The drawing under review shows one solid part. Ordinate dimensions are in mm from its lowest x, y, z. Round coordinates to 2 decimals unless told otherwise and drop trailing zeros. Order: outer loops, then holes, each group sorted by start corner. A loop starts at its lowest first (then second) coordinate and runs counter-clockwise, first axis right, second up. Notation, with made-up numbers: M -35,-17.5 L -15,-17.5 A10 ccw -15,-12.5 Z; hole C -5,78.25 d5. An arc over 180 degrees is marked long. Use a Markdown table: item, result.
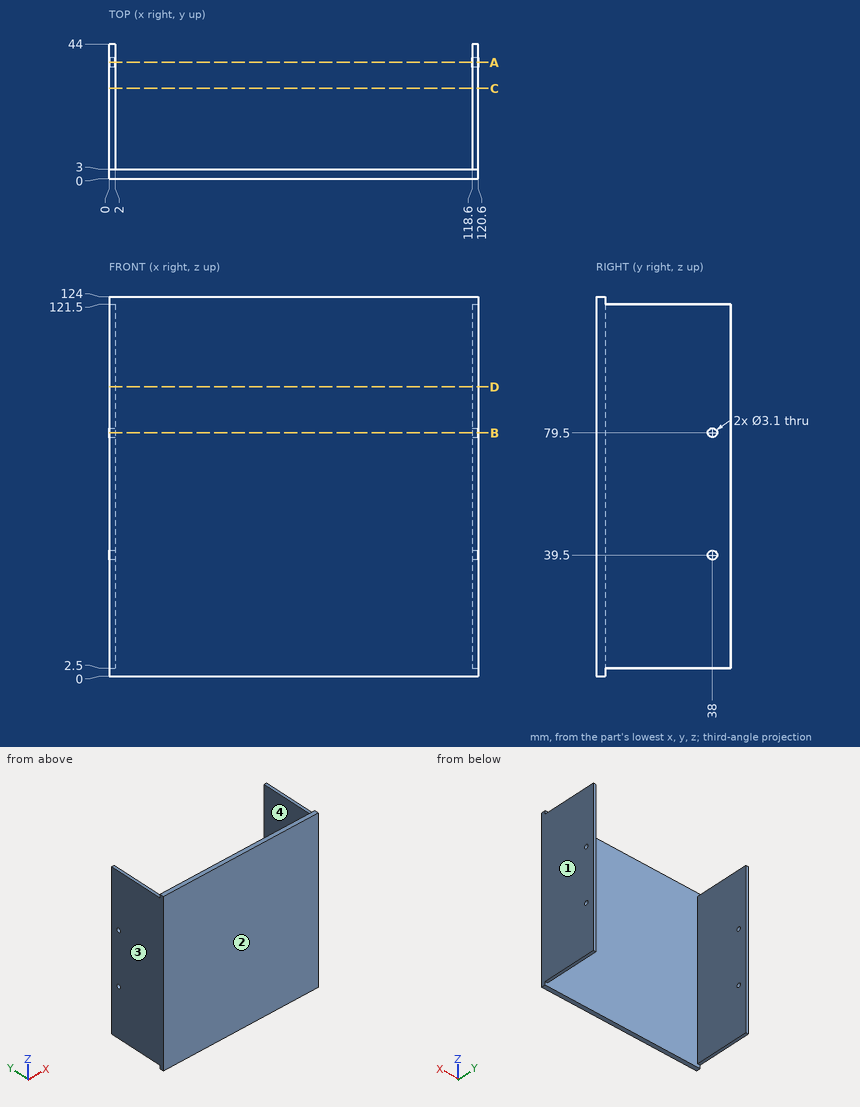
Q1. Wall thickness on line 1 along X through (y, z) = (28, 50); line 2 along Y through (x, z) = (0.65, 39.5); line 3 along Y through (x, z) = (51, 29): over which ranges is each line inside the solid? List them lowest first. Write a range as [from, to].
Determined:
| item | result |
|---|---|
| line 1 | x = [0, 2], [118.6, 120.6] |
| line 2 | y = [0, 36.45], [39.55, 44] |
| line 3 | y = [0, 3] |
Q2. Clearance check with flat-ended pins moving along their axes: pin 1 (2.5 mm diameter, centred on y = 38, z = 79.5, fed in from +X); pin 2 (1 mm diameter, centred on x = 120, y = 31.5, fed in from +Z); pin 3 (2 mm diameter, centred on x = 120, y = 32.5, fed in from -Z). State where each tip first meets the part, or that it passes through.
Determined:
| item | result |
|---|---|
| pin 1 | passes through |
| pin 2 | stops at z = 121.5 |
| pin 3 | stops at z = 2.5 |
Q3. Add section D-D (z = 94.5). Write out the cut boundary in (x, y).
Determined:
| item | result |
|---|---|
| outline | M 0,0 L 120.6,0 L 120.6,44 L 118.6,44 L 118.6,3 L 2,3 L 2,44 L 0,44 Z |
Q4. Draft analysis for pull direction X (two halves, no side actions). For the marked faces 1, 2, 3 and 4, state which applies: pulls with the +X half, pulls with the -X half, needs draft (parallel to the pull), parting line crosses it, or undercut.
Determined:
| item | result |
|---|---|
| face 1 | pulls with the +X half |
| face 2 | needs draft |
| face 3 | pulls with the -X half |
| face 4 | undercut |
Q5. Add section B-B (z = 79.5). Write out the cut boundary in (x, y).
Determined:
| item | result |
|---|---|
| outline | M 0,0 L 120.6,0 L 120.6,36.45 L 118.6,36.45 L 118.6,3 L 2,3 L 2,36.45 L 0,36.45 Z; M 0,39.55 L 2,39.55 L 2,44 L 0,44 Z; M 118.6,39.55 L 120.6,39.55 L 120.6,44 L 118.6,44 Z |
Q6. Add section C-C (y = 29.5). Write out the cut boundary in (x, z).
Determined:
| item | result |
|---|---|
| outline | M 0,2.5 L 2,2.5 L 2,121.5 L 0,121.5 Z; M 118.6,2.5 L 120.6,2.5 L 120.6,121.5 L 118.6,121.5 Z |
Q7. Add section A-A (y = 38). Write out the cut boundary in (x, z).
Determined:
| item | result |
|---|---|
| outline | M 0,2.5 L 2,2.5 L 2,37.95 L 0,37.95 Z; M 0,41.05 L 2,41.05 L 2,77.95 L 0,77.95 Z; M 0,81.05 L 2,81.05 L 2,121.5 L 0,121.5 Z; M 118.6,2.5 L 120.6,2.5 L 120.6,37.95 L 118.6,37.95 Z; M 118.6,41.05 L 120.6,41.05 L 120.6,77.95 L 118.6,77.95 Z; M 118.6,81.05 L 120.6,81.05 L 120.6,121.5 L 118.6,121.5 Z |
